from build123d import *

# Parameters (mm, degrees)
F0_R     = 5
F1_DEPTH = 5
F2_R     = 1
F3_DEPTH = 1


with BuildPart() as f1:
    # F0 (on Front) → F1 (new body)
    with BuildSketch(Plane.XZ):
        with BuildLine():
            ThreePointArc((19.894917, -2.04751), (19.973712, -1.025102), (20, 0))
            ThreePointArc((20, 0), (19.973712, 1.025102), (19.894917, 2.04751))
            ThreePointArc((19.894917, 2.04751), (19.753767, 3.128689), (19.553905, 4.20057))
            ThreePointArc((19.553905, 4.20057), (19.02113, 6.18034), (18.288475, 8.095165))
            ThreePointArc((18.288475, 8.095165), (17.82013, 9.07981), (17.298822, 10.037468))
            ThreePointArc((17.298822, 10.037468), (16.18034, 11.755705), (14.891829, 13.350409))
            ThreePointArc((14.891829, 13.350409), (14.142136, 14.142136), (13.350409, 14.891829))
            ThreePointArc((13.350409, 14.891829), (11.755705, 16.18034), (10.037468, 17.298822))
            ThreePointArc((10.037468, 17.298822), (9.07981, 17.82013), (8.095165, 18.288475))
            ThreePointArc((8.095165, 18.288475), (6.18034, 19.02113), (4.20057, 19.553905))
            ThreePointArc((4.20057, 19.553905), (3.128689, 19.753767), (2.04751, 19.894917))
            ThreePointArc((2.04751, 19.894917), (0, 20), (-2.04751, 19.894917))
            ThreePointArc((-2.04751, 19.894917), (-3.128689, 19.753767), (-4.20057, 19.553905))
            ThreePointArc((-4.20057, 19.553905), (-6.18034, 19.02113), (-8.095165, 18.288475))
            ThreePointArc((-8.095165, 18.288475), (-9.07981, 17.82013), (-10.037468, 17.298822))
            ThreePointArc((-10.037468, 17.298822), (-11.755705, 16.18034), (-13.350409, 14.891829))
            ThreePointArc((-13.350409, 14.891829), (-14.142136, 14.142136), (-14.891829, 13.350409))
            ThreePointArc((-14.891829, 13.350409), (-16.18034, 11.755705), (-17.298822, 10.037468))
            ThreePointArc((-17.298822, 10.037468), (-17.82013, 9.07981), (-18.288475, 8.095165))
            ThreePointArc((-18.288475, 8.095165), (-19.02113, 6.18034), (-19.553905, 4.20057))
            ThreePointArc((-19.553905, 4.20057), (-19.753767, 3.128689), (-19.894917, 2.04751))
            ThreePointArc((-19.894917, 2.04751), (-20, 0), (-19.894917, -2.04751))
            ThreePointArc((-19.894917, -2.04751), (-19.753767, -3.128689), (-19.553905, -4.20057))
            ThreePointArc((-19.553905, -4.20057), (-19.02113, -6.18034), (-18.288475, -8.095165))
            ThreePointArc((-18.288475, -8.095165), (-17.82013, -9.07981), (-17.298822, -10.037468))
            ThreePointArc((-17.298822, -10.037468), (-16.18034, -11.755705), (-14.891829, -13.350409))
            ThreePointArc((-14.891829, -13.350409), (-14.142136, -14.142136), (-13.350409, -14.891829))
            ThreePointArc((-13.350409, -14.891829), (-11.755705, -16.18034), (-10.037468, -17.298822))
            ThreePointArc((-10.037468, -17.298822), (-9.07981, -17.82013), (-8.095165, -18.288475))
            ThreePointArc((-8.095165, -18.288475), (-6.18034, -19.02113), (-4.20057, -19.553905))
            ThreePointArc((-4.20057, -19.553905), (-3.128689, -19.753767), (-2.04751, -19.894917))
            ThreePointArc((-2.04751, -19.894917), (0, -20), (2.04751, -19.894917))
            ThreePointArc((2.04751, -19.894917), (3.128689, -19.753767), (4.20057, -19.553905))
            ThreePointArc((4.20057, -19.553905), (6.18034, -19.02113), (8.095165, -18.288475))
            ThreePointArc((8.095165, -18.288475), (9.07981, -17.82013), (10.037468, -17.298822))
            ThreePointArc((10.037468, -17.298822), (11.755705, -16.18034), (13.350409, -14.891829))
            ThreePointArc((13.350409, -14.891829), (14.142136, -14.142136), (14.891829, -13.350409))
            ThreePointArc((14.891829, -13.350409), (16.18034, -11.755705), (17.298822, -10.037468))
            ThreePointArc((17.298822, -10.037468), (17.82013, -9.07981), (18.288475, -8.095165))
            ThreePointArc((18.288475, -8.095165), (19.02113, -6.18034), (19.553905, -4.20057))
            ThreePointArc((19.553905, -4.20057), (19.753767, -3.128689), (19.894917, -2.04751))
        make_face()
        Circle(F0_R, mode=Mode.SUBTRACT)
        with BuildLine():
            ThreePointArc((19.894917, 2.04751), (19.973712, 1.025102), (20, 0))
            ThreePointArc((20, 0), (19.973712, -1.025102), (19.894917, -2.04751))
            Line((19.894917, -2.04751), (23, -1.5))
            Line((23, -1.5), (23, 0))
            Line((23, 0), (23, 1.5))
            Line((23, 1.5), (19.894917, 2.04751))
        make_face()
        with BuildLine():
            ThreePointArc((18.288475, 8.095165), (19.02113, 6.18034), (19.553905, 4.20057))
            Line((19.553905, 4.20057), (22.337825, 5.680806))
            Line((22.337825, 5.680806), (21.8743, 7.107391))
            Line((21.8743, 7.107391), (21.410774, 8.533976))
            Line((21.410774, 8.533976), (18.288475, 8.095165))
        make_face()
        with BuildLine():
            Line((22.337825, -5.680806), (19.553905, -4.20057))
            ThreePointArc((19.553905, -4.20057), (19.02113, -6.18034), (18.288475, -8.095165))
            Line((18.288475, -8.095165), (21.410774, -8.533976))
            Line((21.410774, -8.533976), (21.8743, -7.107391))
            Line((21.8743, -7.107391), (22.337825, -5.680806))
        make_face()
        with BuildLine():
            ThreePointArc((14.891829, 13.350409), (16.18034, 11.755705), (17.298822, 10.037468))
            Line((17.298822, 10.037468), (19.489069, 12.305535))
            Line((19.489069, 12.305535), (18.607391, 13.519061))
            Line((18.607391, 13.519061), (17.725713, 14.732586))
            Line((17.725713, 14.732586), (14.891829, 13.350409))
        make_face()
        with BuildLine():
            Line((19.489069, -12.305535), (17.298822, -10.037468))
            ThreePointArc((17.298822, -10.037468), (16.18034, -11.755705), (14.891829, -13.350409))
            Line((14.891829, -13.350409), (17.725713, -14.732586))
            Line((17.725713, -14.732586), (18.607391, -13.519061))
            Line((18.607391, -13.519061), (19.489069, -12.305535))
        make_face()
        with BuildLine():
            ThreePointArc((10.037468, 17.298822), (11.755705, 16.18034), (13.350409, 14.891829))
            Line((13.350409, 14.891829), (14.732586, 17.725713))
            Line((14.732586, 17.725713), (13.519061, 18.607391))
            Line((13.519061, 18.607391), (12.305535, 19.489069))
            Line((12.305535, 19.489069), (10.037468, 17.298822))
        make_face()
        with BuildLine():
            Line((14.732586, -17.725713), (13.350409, -14.891829))
            ThreePointArc((13.350409, -14.891829), (11.755705, -16.18034), (10.037468, -17.298822))
            Line((10.037468, -17.298822), (12.305535, -19.489069))
            Line((12.305535, -19.489069), (13.519061, -18.607391))
            Line((13.519061, -18.607391), (14.732586, -17.725713))
        make_face()
        with BuildLine():
            ThreePointArc((4.20057, 19.553905), (6.18034, 19.02113), (8.095165, 18.288475))
            Line((8.095165, 18.288475), (8.533976, 21.410774))
            Line((8.533976, 21.410774), (7.107391, 21.8743))
            Line((7.107391, 21.8743), (5.680806, 22.337825))
            Line((5.680806, 22.337825), (4.20057, 19.553905))
        make_face()
        with BuildLine():
            Line((8.533976, -21.410774), (8.095165, -18.288475))
            ThreePointArc((8.095165, -18.288475), (6.18034, -19.02113), (4.20057, -19.553905))
            Line((4.20057, -19.553905), (5.680806, -22.337825))
            Line((5.680806, -22.337825), (7.107391, -21.8743))
            Line((7.107391, -21.8743), (8.533976, -21.410774))
        make_face()
        with BuildLine():
            ThreePointArc((-2.04751, 19.894917), (0, 20), (2.04751, 19.894917))
            Line((2.04751, 19.894917), (1.5, 23))
            Line((1.5, 23), (0, 23))
            Line((0, 23), (-1.5, 23))
            Line((-1.5, 23), (-2.04751, 19.894917))
        make_face()
        with BuildLine():
            Line((1.5, -23), (2.04751, -19.894917))
            ThreePointArc((2.04751, -19.894917), (0, -20), (-2.04751, -19.894917))
            Line((-2.04751, -19.894917), (-1.5, -23))
            Line((-1.5, -23), (0, -23))
            Line((0, -23), (1.5, -23))
        make_face()
        with BuildLine():
            ThreePointArc((-8.095165, 18.288475), (-6.18034, 19.02113), (-4.20057, 19.553905))
            Line((-4.20057, 19.553905), (-5.680806, 22.337825))
            Line((-5.680806, 22.337825), (-7.107391, 21.8743))
            Line((-7.107391, 21.8743), (-8.533976, 21.410774))
            Line((-8.533976, 21.410774), (-8.095165, 18.288475))
        make_face()
        with BuildLine():
            Line((-5.680806, -22.337825), (-4.20057, -19.553905))
            ThreePointArc((-4.20057, -19.553905), (-6.18034, -19.02113), (-8.095165, -18.288475))
            Line((-8.095165, -18.288475), (-8.533976, -21.410774))
            Line((-8.533976, -21.410774), (-7.107391, -21.8743))
            Line((-7.107391, -21.8743), (-5.680806, -22.337825))
        make_face()
        with BuildLine():
            ThreePointArc((-13.350409, 14.891829), (-11.755705, 16.18034), (-10.037468, 17.298822))
            Line((-10.037468, 17.298822), (-12.305535, 19.489069))
            Line((-12.305535, 19.489069), (-13.519061, 18.607391))
            Line((-13.519061, 18.607391), (-14.732586, 17.725713))
            Line((-14.732586, 17.725713), (-13.350409, 14.891829))
        make_face()
        with BuildLine():
            Line((-12.305535, -19.489069), (-10.037468, -17.298822))
            ThreePointArc((-10.037468, -17.298822), (-11.755705, -16.18034), (-13.350409, -14.891829))
            Line((-13.350409, -14.891829), (-14.732586, -17.725713))
            Line((-14.732586, -17.725713), (-13.519061, -18.607391))
            Line((-13.519061, -18.607391), (-12.305535, -19.489069))
        make_face()
        with BuildLine():
            ThreePointArc((-17.298822, 10.037468), (-16.18034, 11.755705), (-14.891829, 13.350409))
            Line((-14.891829, 13.350409), (-17.725713, 14.732586))
            Line((-17.725713, 14.732586), (-18.607391, 13.519061))
            Line((-18.607391, 13.519061), (-19.489069, 12.305535))
            Line((-19.489069, 12.305535), (-17.298822, 10.037468))
        make_face()
        with BuildLine():
            Line((-17.725713, -14.732586), (-14.891829, -13.350409))
            ThreePointArc((-14.891829, -13.350409), (-16.18034, -11.755705), (-17.298822, -10.037468))
            Line((-17.298822, -10.037468), (-19.489069, -12.305535))
            Line((-19.489069, -12.305535), (-18.607391, -13.519061))
            Line((-18.607391, -13.519061), (-17.725713, -14.732586))
        make_face()
        with BuildLine():
            ThreePointArc((-19.553905, 4.20057), (-19.02113, 6.18034), (-18.288475, 8.095165))
            Line((-18.288475, 8.095165), (-21.410774, 8.533976))
            Line((-21.410774, 8.533976), (-21.8743, 7.107391))
            Line((-21.8743, 7.107391), (-22.337825, 5.680806))
            Line((-22.337825, 5.680806), (-19.553905, 4.20057))
        make_face()
        with BuildLine():
            Line((-21.410774, -8.533976), (-18.288475, -8.095165))
            ThreePointArc((-18.288475, -8.095165), (-19.02113, -6.18034), (-19.553905, -4.20057))
            Line((-19.553905, -4.20057), (-22.337825, -5.680806))
            Line((-22.337825, -5.680806), (-21.8743, -7.107391))
            Line((-21.8743, -7.107391), (-21.410774, -8.533976))
        make_face()
        with BuildLine():
            ThreePointArc((-19.894917, -2.04751), (-20, 0), (-19.894917, 2.04751))
            Line((-19.894917, 2.04751), (-23, 1.5))
            Line((-23, 1.5), (-23, 0))
            Line((-23, 0), (-23, -1.5))
            Line((-23, -1.5), (-19.894917, -2.04751))
        make_face()
    extrude(amount=F1_DEPTH)

    # F2 (on face) → F3 (join)
    with BuildSketch(Plane.XZ.offset(5)):
        with Locations((0, 8)):
            Circle(F2_R)
    extrude(amount=F3_DEPTH)


solid = f1.part
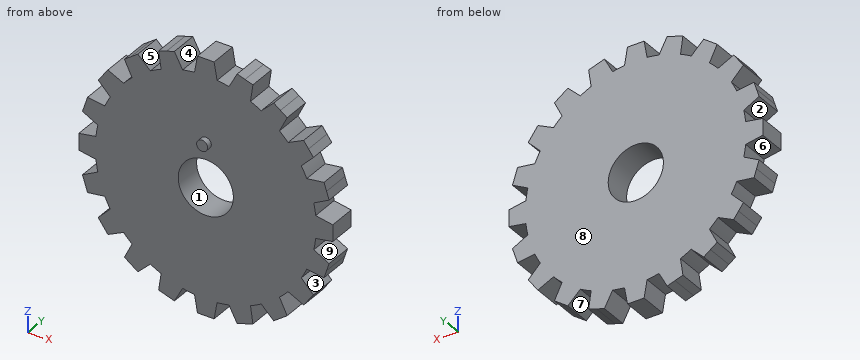
Part model, mm, in its own coordinate system. Face numbers are marked on the shaded views. A direction names the side the tool comes from. Round coordinates to 2 decimals unless told otherwise and drop trailing zeros. Write each loop counter-clockwise with the first axis right and the second up, starting at its lowest first coordinate (ties: lowest second). Pieces come first, ordered by that corner, then holes. Notation, with made-up numbers: (33.5, 43) - (81.5, 43) arc R13 cw to (81.5, 49) - close; hole circle Ø8 at (25.5, -32). An arc over 180 degrees is marked (long way). Use CSV: the item, a comma, the result in double quotes.
Item 1: Slice it at C-C, the plane x = -11. Write the cut outline in (y, z).
Results list:
outline,"(-5, -18.23) - (0, -18.23) - (0, 18.23) - (-5, 18.23) - close"
Item 2: Slice it at B-B, the plane x = 0. Write the cut outline in (y, z), then the cut area to 3 significant figures.
Results list:
outline,"(-6, 7) - (-5, 7) - (-5, 5) - (0, 5) - (0, 23) - (-5, 23) - (-5, 9) - (-6, 9) - close; (-5, -23) - (0, -23) - (0, -5) - (-5, -5) - close"
area,"182 mm²"
Item 3: Wall check: L1, parallel to Z at x = 0, y = -2.85; L2, parallel to X at y = -2.1, z = -20.5; L3, parallel to X at y = -4.6, z = 20. Give the ranges that are in metal, low to high.
Results list:
L1,"z = -23 to -5, 5 to 23"
L2,"x = -8.41 to -4.7, -1.94 to 1.94, 4.7 to 8.41"
L3,"x = -8.34 to -4.44, -2.03 to 2.03, 4.44 to 8.34"
Item 4: Tool access for the marked faces 5, 6, 7, 8 and 9: list every direction of +Z, -Z, +X, -X, +Y, -Y with a clear straight run to the whole face (end or side of a thin tool).
Results list:
face 5,"+Z, +Y, -Y"
face 6,"-X, +Y, -Y"
face 7,"-Z, +Y, -Y"
face 8,"+Z, -Z, +X, -X, +Y"
face 9,"+X, +Y, -Y"
Item 5: Flat gauge pins, fed straight in: P1, Ø1.5, axis at x = 5, y = -2, coming from the +Z side; P2, Ø2, axis at x = -18.5, y = -0.5, coming from the +Z side; P3, Ø5, axis at x = -13, z = 4.5, coming from the +Y side; P4, Ø13, axis at x = 0, z = 0, coming from the -Y side. Where does each tip first touch, or does it go through?
Results list:
P1,"stops at z = 22.34"
P2,"stops at z = 14.73"
P3,"stops at y = 0"
P4,"stops at y = -5"
Item 6: Slice it at A-A, the plane z = 0. Write the cut outline in (x, y).
Results list:
outline,"(-23, -5) - (-5, -5) - (-5, 0) - (-23, 0) - close; (5, -5) - (23, -5) - (23, 0) - (5, 0) - close"
Item 7: Pull direction X, two halves, no side cores. Call the marked faces 1, 2, 3 and 4: pulls with the +X half, pulls with the -X half, needs draft (parallel to the pull), parting line crosses it, or undercut.
Results list:
face 1,"undercut"
face 2,"pulls with the -X half"
face 3,"pulls with the +X half"
face 4,"undercut"
